```python
from build123d import *

# Parameters (mm, degrees)
F0_W          = 61.110928
F0_H          = 56.300208
F1_DEPTH      = 37.51986
F1_DEPTH_BACK = 32.21742
F2_W          = 45.738346
F2_H          = 41.101918
F3_DEPTH      = 7.84984
F4_W          = 30.494862
F4_H          = 26.376776
F5_DEPTH      = 4.4368


with BuildPart() as f1:
    # F0 (on Top) → F1 (new body, two sides)
    with BuildSketch(Plane.XY) as f1_sk:
        Rectangle(F0_W, F0_H)
    extrude(amount=F1_DEPTH)
    extrude(f1_sk.sketch, amount=-F1_DEPTH_BACK)

    # F2 (on face) → F3 (join)
    with BuildSketch(Plane.XY.offset(37.51986)):
        Rectangle(F2_W, F2_H)
    extrude(amount=F3_DEPTH)

    # F4 (on face) → F5 (join)
    with BuildSketch(Plane.XY.offset(45.3697)):
        Rectangle(F4_W, F4_H)
    extrude(amount=F5_DEPTH)


solid = f1.part
```
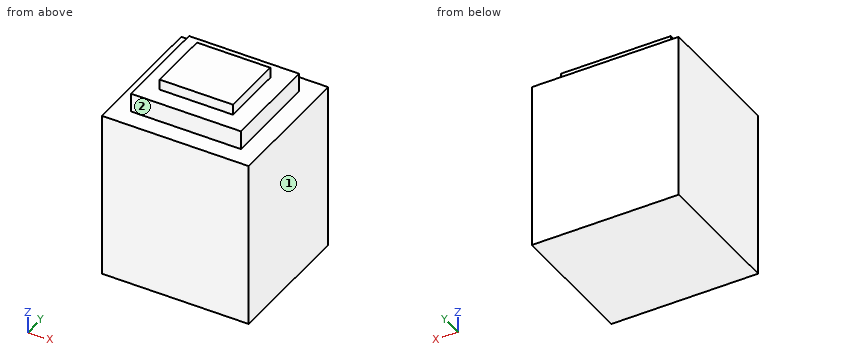
Work out the finished part from the listing and answer in its coordinate system (mm). Face numbers are marked on the shaded views. A direction names the side the tool comes from. Give positions to 0.01 mm unless a question says otherwise; leave off trailing zeros. Loops run counter-clockwise (first coordinate to the right, second up) from the corner with the lowest first, then second, coordinate; pieces in that order, holes last. Notation, with made-up numbers: (47.5, 56) -> (95.5, 56) arc R21 cw to (95.5, 78) -> close; hole circle Ø3 at (60, 87). An arc over 180 degrees is marked (long way). Put each result on its own line as item: value. Start each with the question number.
Item 1: Find the intervals of material crossed by L1, parallel to Y at x = -8, z = 46; L2, parallel to Z at x = -8, y = 24; L3, parallel to Z at x = -8, y = -17.5, in increasing order. Write a range as [from, to].
Item 2: The part is cut by section C-C (z = 43). Give the vertices of the cut face in (x, y).
Item 3: Which of the six approach directions +Z, -Z, +X, -X, +Y, -Y give full straight-line access (tool end or side, diameter ignored) to the marked faces 1 and 2?
Item 4: The part is cut by section D-D (y = 19). Give the vertices of the cut face in (x, z), then the cut area to 3 significant figures.
Item 5: Each of these flat-tipped pins is pushed along its axis until it touches: P1, Ø2.5, axis at x = -11.5, z = 41, coming from the +Y side; P2, Ø2, axis at x = -4.5, z = 47.5, coming from the -Y side; P3, Ø4, axis at y = -2.5, z = 42, coming from the +X side. Where does it stop, or does it pass through?
Item 6: The part is cut by section B-B (x = -12). Give the vertices of the cut face in (y, z), then the cut area to 3 significant figures.
Item 7: The part is cut by section A-A (y = 0). Give the vertices of the cut face in (x, z), then the cut area to 3 significant figures.
Answers below:
1. L1: [-13.19, 13.19]
1. L2: [-32.22, 37.52]
1. L3: [-32.22, 45.37]
2. outline: (-22.87, -20.55) -> (22.87, -20.55) -> (22.87, 20.55) -> (-22.87, 20.55) -> close
3. face 1: +Z, -Z, +X, +Y, -Y
3. face 2: +Z, +X, -X, -Y
4. outline: (-30.56, -32.22) -> (30.56, -32.22) -> (30.56, 37.52) -> (22.87, 37.52) -> (22.87, 45.37) -> (-22.87, 45.37) -> (-22.87, 37.52) -> (-30.56, 37.52) -> close
4. area: 4,620 mm2
5. P1: y = 20.55
5. P2: y = -13.19
5. P3: x = 22.87
6. outline: (-28.15, -32.22) -> (28.15, -32.22) -> (28.15, 37.52) -> (20.55, 37.52) -> (20.55, 45.37) -> (13.19, 45.37) -> (13.19, 49.81) -> (-13.19, 49.81) -> (-13.19, 45.37) -> (-20.55, 45.37) -> (-20.55, 37.52) -> (-28.15, 37.52) -> close
6. area: 4,370 mm2
7. outline: (-30.56, -32.22) -> (30.56, -32.22) -> (30.56, 37.52) -> (22.87, 37.52) -> (22.87, 45.37) -> (15.25, 45.37) -> (15.25, 49.81) -> (-15.25, 49.81) -> (-15.25, 45.37) -> (-22.87, 45.37) -> (-22.87, 37.52) -> (-30.56, 37.52) -> close
7. area: 4,760 mm2
